from build123d import *

# Parameters (mm, degrees)
F0_W        = 7
F0_H        = 5
F1_DEPTH    = 4
F2_T1_DEPTH = 4
F2_T3_DEPTH = 14


# Not quite as in the source:
# - a fillet or chamfer that OpenCascade refuses, or shapes differently, is made with other operations: its cross-section is extruded or revolved along the edge and cut away or added
# - a feature names something its author has since deleted; it is built from what else it names


with BuildPart() as f1:
    # F0 (on Top) → F1 (new body)
    with BuildSketch(Plane.XY):
        with BuildLine():
            Line((-51, 139), (-51, -4))
            Line((-51, -4), (69.5775999523, -4))
            Line((69.5775999523, -4), (69.5775999523, 0))
            Line((69.5775999523, 0), (66.3850666349, 0))
            Line((66.3850666349, 0), (46.3850666349, 0))
            Line((46.3850666349, 0), (43.1925333174, 0))
            Line((43.1925333174, 0), (23.1925333174, 0))
            Line((23.1925333174, 0), (20, 0))
            Line((20, 0), (0, 0))
            Line((0, 0), (-44.4302483166, 139.9080159757))
            ThreePointArc((-44.4302483166, 139.9080159757), (-45.5180993372, 141.4211616971), (-47.2895326655, 142))
            Line((-47.2895326655, 142), (-48, 142))
            ThreePointArc((-48, 142), (-50.1213203436, 141.1213203436), (-51, 139))
        make_face()
        with Locations((-40.5, 2.5)):
            Rectangle(F0_W, F0_H, mode=Mode.SUBTRACT)
        with Locations((-26.5, 2.5)):
            Rectangle(F0_W, F0_H, mode=Mode.SUBTRACT)
        with Locations((-12.5, 2.5)):
            Rectangle(F0_W, F0_H, mode=Mode.SUBTRACT)
        with BuildLine():
            Line((-7.3725300405, 9), (-47, 9))
            ThreePointArc((-47, 9), (-47.7071067812, 9.2928932188), (-48, 10))
            Line((-48, 10), (-48, 71.4074290533))
            ThreePointArc((-48, 71.4074290533), (-47.7071067812, 72.1145358345), (-47, 72.4074290533))
            Line((-47, 72.4074290533), (-26.8735379155, 72.4074290533))
            ThreePointArc((-26.8735379155, 72.4074290533), (-26.2830601394, 72.2144829523), (-25.9204431326, 71.7101010452))
            Line((-25.9204431326, 71.7101010452), (-6.4194352575, 10.3026719919))
            ThreePointArc((-6.4194352575, 10.3026719919), (-6.5654761415, 9.4095222239), (-7.3725300405, 9))
        make_face(mode=Mode.SUBTRACT)
        with Locations((-37.5, 76.9074290533)):
            Rectangle(F0_W, F0_H, mode=Mode.SUBTRACT)
        with BuildLine():
            ThreePointArc((-48, 134.7843734895), (-47.1531424452, 135.7725776139), (-46.046905217, 135.0870454814))
            Line((-46.046905217, 135.0870454814), (-29.4136863758, 82.7101010452))
            ThreePointArc((-29.4136863758, 82.7101010452), (-29.5597272597, 81.8169512772), (-30.3667811588, 81.4074290533))
            Line((-30.3667811588, 81.4074290533), (-47, 81.4074290533))
            ThreePointArc((-47, 81.4074290533), (-47.7071067812, 81.7003222721), (-48, 82.4074290533))
            Line((-48, 82.4074290533), (-48, 134.7843734895))
        make_face(mode=Mode.SUBTRACT)
        Polygon((66.3850666349, 0), (69.5775999523, 0), (65.783943064, 10.4229866378), (62.9648652016, 9.3969262079), align=None)
        Polygon((43.1925333174, 0), (46.3850666349, 0), (42.5914097465, 10.4229866378), (39.7723318842, 9.3969262079), align=None)
        Polygon((16.5797985667, 9.3969262079), (20, 0), (23.1925333174, 0), (19.3988764291, 10.4229866378), align=None)
    extrude(amount=F1_DEPTH)

    # F2: fillet of radius 2 on 14 edges, made by hand

    # F2_s2 → F2_t1 (join)
    with BuildSketch(Plane.XY):
        with BuildLine():
            ThreePointArc((42.2156225455, 2.6840402867), (41.9745413925, 0.8528471273), (40.3362373039, 0))
            Line((40.3362373039, 0), (43.1925333174, 0))
            Line((43.1925333174, 0), (42.2156225455, 2.6840402867))
        make_face()
        with BuildLine():
            ThreePointArc((47.7854817113, 0), (46.6383288386, 0.3616959114), (45.9060964697, 1.3159597133))
            Line((45.9060964697, 1.3159597133), (46.3850666349, 0))
            Line((46.3850666349, 0), (47.7854817113, 0))
        make_face()
        with BuildLine():
            ThreePointArc((65.4081558629, 2.6840402867), (65.1670747099, 0.8528471273), (63.5287706214, 0))
            Line((63.5287706214, 0), (66.3850666349, 0))
            Line((66.3850666349, 0), (65.4081558629, 2.6840402867))
        make_face()
        with BuildLine():
            ThreePointArc((24.5929483938, 0), (23.4457955211, 0.3616959114), (22.7135631523, 1.3159597133))
            Line((22.7135631523, 1.3159597133), (23.1925333174, 0))
            Line((23.1925333174, 0), (24.5929483938, 0))
        make_face()
        with BuildLine():
            ThreePointArc((19.0230892281, 2.6840402867), (18.7820080751, 0.8528471273), (17.1437039865, 0))
            Line((17.1437039865, 0), (20, 0))
            Line((20, 0), (19.0230892281, 2.6840402867))
        make_face()
        with BuildLine():
            ThreePointArc((1.4632920473, 0), (0.2823364951, 0.3858922019), (-0.4428975187, 1.3946560162))
            Line((-0.4428975187, 1.3946560162), (0, 0))
            Line((0, 0), (1.4632920473, 0))
        make_face()
    extrude(amount=F2_T1_DEPTH)

    # F2_s4 → F2_t3 (cut)
    with BuildSketch(Plane.XY.offset(-5)):
        with BuildLine():
            ThreePointArc((66.4679833506, 8.5436013963), (65.4338346325, 9.6721766837), (63.9045578224, 9.7389463512))
            Line((63.9045578224, 9.7389463512), (65.783943064, 10.4229866378))
            Line((65.783943064, 10.4229866378), (66.4679833506, 8.5436013963))
        make_face()
        with BuildLine():
            ThreePointArc((64.8442504432, 10.0809664945), (63.7156751557, 9.0468177764), (63.6489054883, 7.5175409663))
            Line((63.6489054883, 7.5175409663), (62.9648652016, 9.3969262079))
            Line((62.9648652016, 9.3969262079), (64.8442504432, 10.0809664945))
        make_face()
        with BuildLine():
            ThreePointArc((20.0829167158, 8.5436013963), (19.0487679977, 9.6721766837), (17.5194911875, 9.7389463512))
            Line((17.5194911875, 9.7389463512), (19.3988764291, 10.4229866378))
            Line((19.3988764291, 10.4229866378), (20.0829167158, 8.5436013963))
        make_face()
        with BuildLine():
            ThreePointArc((18.4591838083, 10.0809664945), (17.3306085209, 9.0468177764), (17.2638388534, 7.5175409663))
            Line((17.2638388534, 7.5175409663), (16.5797985667, 9.3969262079))
            Line((16.5797985667, 9.3969262079), (18.4591838083, 10.0809664945))
        make_face()
        with BuildLine():
            ThreePointArc((41.6517171257, 10.0809664945), (40.5231418383, 9.0468177764), (40.4563721708, 7.5175409663))
            Line((40.4563721708, 7.5175409663), (39.7723318842, 9.3969262079))
            Line((39.7723318842, 9.3969262079), (41.6517171257, 10.0809664945))
        make_face()
        with BuildLine():
            ThreePointArc((43.2754500332, 8.5436013963), (42.2413013151, 9.6721766837), (40.712024505, 9.7389463512))
            Line((40.712024505, 9.7389463512), (42.5914097465, 10.4229866378))
            Line((42.5914097465, 10.4229866378), (43.2754500332, 8.5436013963))
        make_face()
        with BuildLine():
            ThreePointArc((67.5775999523, -4), (68.9918135147, -3.4142135624), (69.5775999523, -2))
            Line((69.5775999523, -2), (69.5775999523, -4))
            Line((69.5775999523, -4), (67.5775999523, -4))
        make_face()
        with BuildLine():
            ThreePointArc((-51, -2), (-50.4142135624, -3.4142135624), (-49, -4))
            Line((-49, -4), (-51, -4))
            Line((-51, -4), (-51, -2))
        make_face()
    extrude(amount=F2_T3_DEPTH, mode=Mode.SUBTRACT)


solid = f1.part
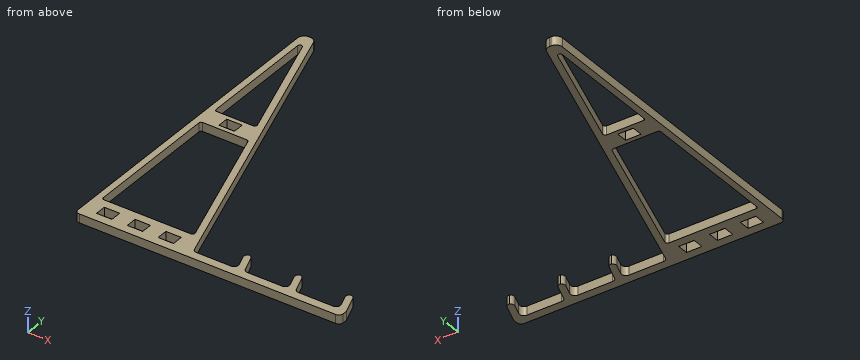
Geometry check sheet. Reference: the model listing, model coordinates, mm. Round coordinates to 2 decimals unless told otherwise and drop trailing zeros. Loops run counter-clockwise (first coordinate to the right, second up) from the corner with the lowest first, then second, coordinate; pieces in that order, holes last. Notation, with made-up numbers: (30, 50.25) - (87, 50.25) arc R26 ccw to (87, 64.25) - close; hole circle Ø6 at (44.5, 63). An arc over 180 degrees is marked (long way). One line per question, with ' | ' between items. Start each with the question number.
1. Depth check by flat-ended pin: pin 1 (2 mm diameter, centred on x = 6.5, z = 1, fed in from +Y); pin 2 (2 mm diameter, centred on y = 116, z = 3.5, fed in from +X). Enter the tip coordinate at first touch or a pass-through.
2. Cross-section at D-D on y = 61. Record the cut outline in (x, z), then the cut area to 3 significant figures.
3. Cross-section at B-B on x = 5.5. Record the cut outline in (y, z).
4. Scan lines: line 1 (Y direction, x = 51, z = 2.85); line 2 (X direction, y = 21, z = 0.8); line 3 (X direction, y = 130, z = 1.8). Record each from-to range of solid material in increasing order. Write a range as [from, to].
5. Cross-section at C-C on z = 2.3. State how many separate pieces and enclosed holes the cut face has, then the cut area to 3 significant figures.
6. Cross-section at A-A on y = 77. Record the cut outline in (x, z), then the cut area to 3 significant figures.
Taken from the geometry:
1) pin 1: y = 0 | pin 2: x = -36.52
2) outline: (-51, 0) - (-48, 0) - (-48, 4) - (-51, 4) - close; (-22.52, 0) - (-19.37, 0) - (-19.37, 4) - (-22.52, 4) - close | area: 24.6 mm²
3) outline: (-4, 0) - (0, 0) - (0, 4) - (-4, 4) - close
4) line 1: [-4, 0] | line 2: [-51, -48], [-9.82, -6.67] | line 3: [-51, -48], [-44.43, -41.28]
5) separate pieces: 1 | enclosed holes: 6 | area: 1,890 mm²
6) outline: (-51, 0) - (-41, 0) - (-41, 4) - (-51, 4) - close; (-34, 0) - (-24.45, 0) - (-24.45, 4) - (-34, 4) - close | area: 78.2 mm²
